Can you work these out from the model? Positions are in its coordinate system, mm. Face numbers are marked on the shaded views. A direction names the side the tool comes from. Coordinates: 2 decimals unless noted, no trailing zeros. Loops run counter-clockwise (first coordinate to the right, second up) from the corner with the lowest first, then second, coordinate; pieces in that order, holes last. Notation, with made-up numbers: (-32, 38) -> (-20, 38) arc R10 ccw to (-20, 43) -> close; hole circle Ø3 at (48.5, 5). An arc over 180 degrees is marked (long way). Put each result on its own line as item: value. Start each with the question number.
Item 1: If we section it at D-D on x = 21: Please give me the cut outline in (y, z), plus the area to 3 significant figures.
Item 2: If we section it at C-C on x = 4: Please give me the cut outline in (y, z), plus the area to 3 significant figures.
Item 3: If we section it at A-A on z = 0: Please give me the cut outline in (x, y).
Item 4: Will these pins go through, and if not, where does the flat tip stop? P1, Ø5, axis at y = 16, z = -12, coming from the -X side; P2, Ø1, axis at y = 5.5, z = -22, coming from the +X side; P3, Ø2.5, axis at x = 2.5, y = 1, coming from the -Z side; P4, Ø1.3, axis at x = -17.06, z = 30.22, coming from the +Y side.
Item 5: If we section it at B-B on z = -18.2: Please give me the cut outline in (x, y).
Item 6: Please list where these lines run through material, in increasing order: L1, parallel to Y at x = -6, z = 27.5; L2, parallel to X at y = 2.5, z = 34; L3, parallel to Y at x = -9.5, z = 15. Write a range as from..to.
Item 7: For the marked faces 1 and 2, which set-ups out of +Z, -Z, +X, -X, +Y, -Y let a thin tool reach every point of the face, with its end or its side?
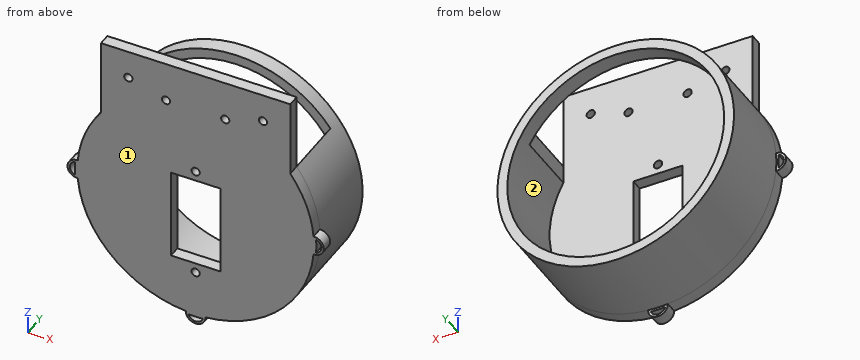
```python
from build123d import *

# Parameters (mm, degrees)
SKETCH1_W           = 12.5
SKETCH1_H           = 23.2
BOSS_EXTRUDE1_DEPTH = 3
SKETCH4_R           = 30
SKETCH4_R_2         = 27.5
BOSS_EXTRUDE3_DEPTH = 20
SKETCH5_R           = 1.05
CUT_EXTRUDE2_DEPTH  = 51.124844139
BOSS_EXTRUDE4_DEPTH = 3
CUT_EXTRUDE11_START = -8.575715
SKETCH9_W           = 48
SKETCH9_H           = 16
CUT_EXTRUDE11_DEPTH = 16.574279
CUT_EXTRUDE12_DEPTH = 52.393398578
BOSS_EXTRUDE8_START = -3
BOSS_EXTRUDE8_DEPTH = 3
SKETCH10_R          = 1.05
CUT_EXTRUDE13_DEPTH = 54.449294936


with BuildPart() as part:
    # Sketch1 → Boss-Extrude1 (new body)
    with BuildSketch(Plane(origin=(0, 0, 0), x_dir=(1, 0, 0), z_dir=(0, 1, 0))):
        with BuildLine():
            ThreePointArc((-29.895833333, -2.497828918), (0, -30), (29.895833333, -2.497828918))
            ThreePointArc((29.895833333, -2.497828918), (32.5, 0), (29.895833333, 2.497828918))
            ThreePointArc((29.895833333, 2.497828918), (21.213203436, 21.213203436), (2.497828918, 29.895833333))
            ThreePointArc((2.497828918, 29.895833333), (0, 32.5), (-2.497828918, 29.895833333))
            ThreePointArc((-2.497828918, 29.895833333), (-21.213203436, 21.213203436), (-29.895833333, 2.497828918))
            ThreePointArc((-29.895833333, 2.497828918), (-32.5, 0), (-29.895833333, -2.497828918))
        make_face()
        with Locations((0, 4.1)):
            Rectangle(SKETCH1_W, SKETCH1_H, mode=Mode.SUBTRACT)
    extrude(amount=BOSS_EXTRUDE1_DEPTH)

    # Sketch4 → Boss-Extrude3 (add)
    with BuildSketch(Plane(origin=(0, 3, 0), x_dir=(1, 0, 0), z_dir=(0, 1, 0))):
        with Locations(Location((0, 0, 0), (0, 0, 85.223969073))):
            Circle(SKETCH4_R)
        with Locations(Location((0, 0, 0), (0, 0, 270))):
            Circle(SKETCH4_R_2, mode=Mode.SUBTRACT)
    extrude(amount=BOSS_EXTRUDE3_DEPTH)

    # Sketch5 → Cut-Extrude2 (cut, through all)
    with BuildSketch(Plane(origin=(0, 3, 0), x_dir=(1, 0, 0), z_dir=(0, 1, 0))):
        with Locations(Location((0, 18.2, 0), (0, 0, 270))):
            Circle(SKETCH5_R)
        with Locations(Location((0, -10, 0), (0, 0, 270))):
            Circle(SKETCH5_R)
    extrude(amount=-CUT_EXTRUDE2_DEPTH, mode=Mode.SUBTRACT)

    # Sketch6 → Boss-Extrude4 (add)
    with BuildSketch(Plane(origin=(0, 0, 0), x_dir=(1, 0, 0), z_dir=(0, 1, 0))):
        with BuildLine():
            Line((-21, -21.424285286), (-21, -34.424285286))
            Line((-21, -34.424285286), (21, -34.424285286))
            Line((21, -34.424285286), (21, -21.424285286))
            ThreePointArc((21, -21.424285286), (0, -30), (-21, -21.424285286))
        make_face()
    extrude(amount=BOSS_EXTRUDE4_DEPTH)

    # Sketch9 → Cut-Extrude11 (cut)
    with BuildSketch(Plane(origin=(0, 0, 21.424285286), x_dir=(-1, 0, 0), z_dir=(0, 0, -1)).offset(CUT_EXTRUDE11_START)):
        with Locations((0, 11)):
            Rectangle(SKETCH9_W, SKETCH9_H)
    extrude(amount=CUT_EXTRUDE11_DEPTH, mode=Mode.SUBTRACT)

    # Sketch12 → Cut-Extrude12 (cut, through all)
    with BuildSketch(Plane(origin=(0, 3, 0), x_dir=(1, 0, 0), z_dir=(0, 1, 0))):
        with BuildLine():
            ThreePointArc((1.819908232, 30.545833333), (0, 30.6), (-1.819908232, 30.545833333))
            ThreePointArc((-1.819908232, 30.545833333), (0, 31.9), (1.819908232, 30.545833333))
        make_face()
        with BuildLine():
            ThreePointArc((30.545833333, -1.819908232), (30.6, 0), (30.545833333, 1.819908232))
            ThreePointArc((30.545833333, 1.819908232), (31.9, 0), (30.545833333, -1.819908232))
        make_face()
        with BuildLine():
            ThreePointArc((-30.545833333, 1.819908232), (-30.6, 0), (-30.545833333, -1.819908232))
            ThreePointArc((-30.545833333, -1.819908232), (-31.9, 0), (-30.545833333, 1.819908232))
        make_face()
    extrude(amount=-CUT_EXTRUDE12_DEPTH, mode=Mode.SUBTRACT)

    # Sketch13 → Boss-Extrude8 (add)
    with BuildSketch(Plane(origin=(0, 3, 0), x_dir=(1, 0, 0), z_dir=(0, 1, 0)).offset(BOSS_EXTRUDE8_START)):
        with BuildLine():
            Line((21, -34.424285286), (21, -21.424285286))
            ThreePointArc((21, -21.424285286), (22.565048913, -19.769131685), (24, -18))
            Line((24, -18), (24, -37.424285286))
            Line((24, -37.424285286), (-24, -37.424285286))
            Line((-24, -37.424285286), (-24, -18))
            ThreePointArc((-24, -18), (-22.565048913, -19.769131685), (-21, -21.424285286))
            Line((-21, -21.424285286), (-21, -34.424285286))
            Line((-21, -34.424285286), (21, -34.424285286))
        make_face()
    extrude(amount=BOSS_EXTRUDE8_DEPTH)

    # Sketch10 → Cut-Extrude13 (cut, through all)
    with BuildSketch(Plane(origin=(0, 3, 0), x_dir=(1, 0, 0), z_dir=(0, 1, 0))):
        with Locations(Location((-7.5, -27.296921086, 0), (0, 0, 270))):
            Circle(SKETCH10_R)
        with Locations(Location((-17.06304756, -30.220638133, 0), (0, 0, 270))):
            Circle(SKETCH10_R)
        with Locations(Location((7.5, -27.296921086, 0), (0, 0, 270))):
            Circle(SKETCH10_R)
        with Locations(Location((17.06304756, -30.220638133, 0), (0, 0, 270))):
            Circle(SKETCH10_R)
    extrude(amount=-CUT_EXTRUDE13_DEPTH, mode=Mode.SUBTRACT)


solid = part.part
```
Solutions:
1. outline: (0, -21.42) -> (23, -21.42) -> (23, -17.76) -> (3, -17.76) -> (3, 37.42) -> (0, 37.42) -> close; (19, 17.76) -> (23, 17.76) -> (23, 21.42) -> (19, 21.42) -> close
1. area: 265 mm^2
2. outline: (0, -29.73) -> (23, -29.73) -> (23, -27.21) -> (3, -27.21) -> (3, -15.7) -> (0, -15.7) -> close; (0, 7.5) -> (3, 7.5) -> (3, 37.42) -> (0, 37.42) -> close; (19, 27.21) -> (23, 27.21) -> (23, 29.73) -> (19, 29.73) -> close
2. area: 192 mm^2
3. outline: (-32.5, 0) -> (-31.9, 0) -> (-31.9, 3) -> (-32.5, 3) -> close; (-30.6, 0) -> (-6.25, 0) -> (-6.25, 3) -> (-27.5, 3) -> (-27.5, 23) -> (-30, 23) -> (-30, 3) -> (-30.6, 3) -> close; (6.25, 0) -> (30.6, 0) -> (30.6, 3) -> (30, 3) -> (30, 23) -> (27.5, 23) -> (27.5, 3) -> (6.25, 3) -> close; (31.9, 0) -> (32.5, 0) -> (32.5, 3) -> (31.9, 3) -> close
4. P1: x = -28.46
4. P2: x = 20.92
4. P3: z = -32.17
4. P4: through
5. outline: (-23.85, 0) -> (-1.05, 0) -> (-1.05, 3) -> (-20.62, 3) -> (-20.62, 23) -> (-23.85, 23) -> close; (1.05, 0) -> (23.85, 0) -> (23.85, 23) -> (20.62, 23) -> (20.62, 3) -> (1.05, 3) -> close
6. L1: 0..3, 19..23
6. L2: -24..24
6. L3: 0..3
7. face 1: +Z, -Z, +X, -X, -Y
7. face 2: +Y
